```python
from build123d import *

# Parameters (mm, degrees)
SKETCH_R     = 5
PAD_DEPTH    = 10
CHAMFER_SIZE = 2
FILLET_R     = 2
FILLET001_R  = 1


with BuildPart() as part:
    # Sketch → Pad (new body)
    with BuildSketch(Plane.XZ):
        with BuildLine():
            Line((0, 35), (50, 35))
            ThreePointArc((50, 35), (54.393398, 24.393398), (65, 20))
            Line((65, 20), (65, 0))
            Line((65, 0), (15, 0))
            ThreePointArc((15, 0), (10.606602, 10.606602), (0, 15))
            Line((0, 15), (0, 35))
        make_face()
        with Locations((10, 25)):
            Circle(SKETCH_R, mode=Mode.SUBTRACT)
        with Locations((55, 10)):
            Circle(SKETCH_R, mode=Mode.SUBTRACT)
    extrude(amount=PAD_DEPTH)

    # Chamfer
    chamfer_edges = [part.edges().sort_by_distance(p)[0] for p in [
        (5, -10, 25),
        (50, -10, 10),
    ]]
    chamfer(chamfer_edges, length=CHAMFER_SIZE)

    # Fillet
    fillet_edges = [part.edges().sort_by_distance(p)[0] for p in [
        (65, -10, 10),
        (40, -10, 0),
        (0, -10, 25),
        (25, -10, 35),
        (54.393398, -10, 24.393398),
        (10.606602, -10, 10.606602),
    ]]
    fillet(fillet_edges, radius=FILLET_R)

    # Fillet001
    fillet001_edges = [part.edges().sort_by_distance(p)[0] for p in [
        (0, -4, 35),
    ]]
    fillet(fillet001_edges, radius=FILLET001_R)


solid = part.part
```
Verification items for the finished model (mm, model axes). Coordinates: 2 decimals unless noted, no trailing zeros. Order: outer loops, then holes, each group sorted by start corner. A loop starts at its lowest first (then second) coordinate and runs counter-clockwise, first axis right, second up. Notation, with made-up numbers: (1, 84) -> (8, 84) arc R13 ccw to (8, 95) -> close; hole circle Ø9 at (43.5, -5). An arc over 180 degrees is marked (long way). Put each result on its own line as item: value. Start each with the question number.
1) Material ranges on L1, parallel to Z at x = 56, y = -3; L2, parallel to X at y = -6, z = 29; L3, parallel to Z at x = 55, y = -5, recorded low to high.
2) Go/stop test with flat-tipped pins: pin 1 (2 mm diameter, centred on x = 24, z = 17, fed in from +Y); pin 2 (5 mm diameter, centred on y = -7.5, z = 5.5, fed in from -X); pin 3 (11.5 mm diameter, centred on x = 55, z = 10, fed in from -Y). Record where each tip stops, or that it passes through.
3) Cross-section at A-A (y = -7). Enter the section's corners in (x, z).
4) Release check for a two-part mould opening along Z. For faces 1 (the cylindrical face through (51, -4, 13)), 2 (the cylindrical face through (0.6, -9.43, 24.63)), 3 (the cylindrical face through (10.72, -3.94, 10.49)) record: pulls with the +Z half, pulls with the -Z half, needs draft (parallel to the pull), parting line crosses it, or undercut.
Geometry check:
1. L1: z = 0 to 5.1, 14.9 to 23
1. L2: x = 0 to 7, 13 to 51.25
1. L3: z = 0 to 5, 15 to 23.82
2. pin 1: stops at y = 0
2. pin 2: stops at x = 12.69
2. pin 3: stops at y = -8.75
3. outline: (0, 15) arc R15 cw to (15, 0) -> (65, 0) -> (65, 20) arc R15 cw to (50, 35) -> (1, 35) arc R1 ccw to (0, 34) -> close; hole circle Ø10 at (10, 25); hole circle Ø10 at (55, 10)
4. face 1: undercut
4. face 2: needs draft
4. face 3: pulls with the -Z half
